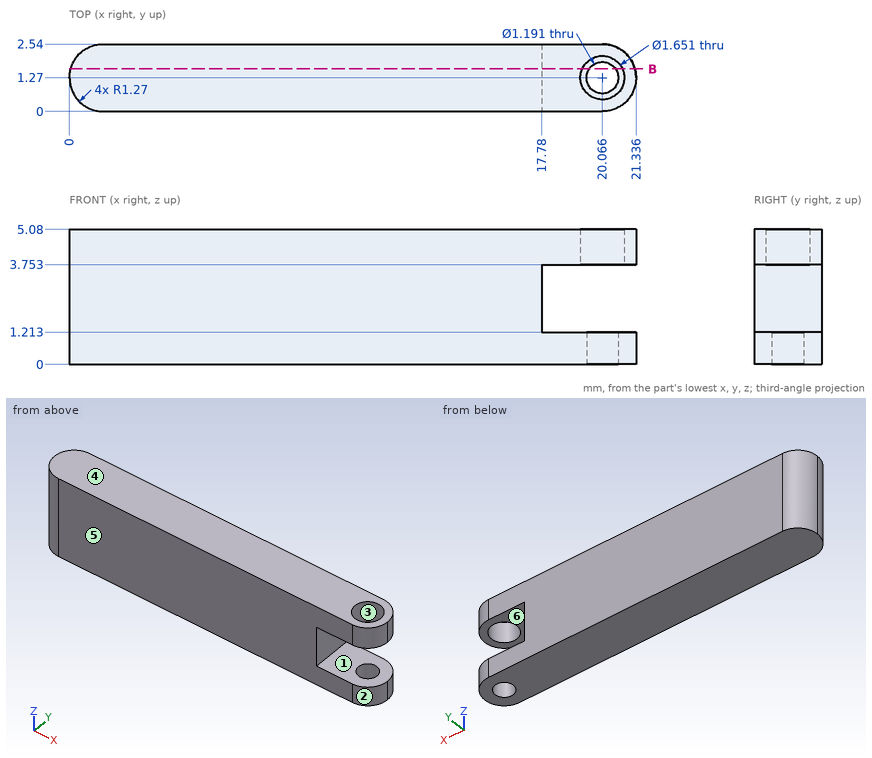
Geometry: see drawing. Coordinates: mm, zero at the bounding-box minimum. A direction names the side the tool comes from. Round coordinates to 2 decimals unless told otherwise and drop trailing zeros. Loops run counter-clockwise (first coordinate to the right, second up) from the corner with the lowest first, then second, coordinate; pieces in that order, holes last. Notation, with made-up numbers: (61, 72.5) -> (92, 72.5) arc R25 cw to (92, 86.5) -> close; hole circle Ø11 at (15, -24). An arc over 180 degrees is marked (long way). Use one line per item in the form item = value. Start each with the question number.
Item 1: Contact query for a flat-ended pin moving along its axis: pin 1 Ø0.8 at (y, z) = (2, 2.5) entering from +X. Output: stop coordinate, or through.
Item 2: Material intervals for L1, parallel to Z at x = 19, y = 0.75; L2, parallel to X at y = 1.35, z = 4.3 (1 decimal); L3, parallel to X at y = 1.7, z = 0.65 (1 decimal), sorted ascending. Write a range as from..to.
Item 3: Set-up query: the marked faces 1, 2 and 3. Return all of +Z, -Z, +X, -X, +Y, -Y with unobstructed straight access to the full face (end or side cutting, diameter ignored); none if empty.
Item 4: Section query B-B on y = 1.6. Return the cut outline in (x, z), then the cut area to 3 significant figures.
Item 5: Mould query, pull axis Z, two halves, no side actions, for the marked faces 4, 5 and 6. Classes: pulls with the +Z half, pulls with the -Z half, needs draft (parallel to the pull), parting line crosses it, or undercut.
Ans:
q1.pin_1 = 17.78
q2.L1 = 0..1.21, 3.75..5.08
q2.L2 = 0..19.2, 20.9..21.3
q2.L3 = 0.1..19.7, 20.5..21.3
q3.face_1 = +X, +Y, -Y
q3.face_2 = +Z, -Z, +X, -Y
q3.face_3 = +Z
q4.outline = (0.04, 0) -> (19.57, 0) -> (19.57, 1.21) -> (17.78, 1.21) -> (17.78, 3.75) -> (19.31, 3.75) -> (19.31, 5.08) -> (0.04, 5.08) -> close; (20.56, 0) -> (21.29, 0) -> (21.29, 1.21) -> (20.56, 1.21) -> close; (20.82, 3.75) -> (21.29, 3.75) -> (21.29, 5.08) -> (20.82, 5.08) -> close
q4.area = 95.8 mm^2
q5.face_4 = pulls with the +Z half
q5.face_5 = needs draft
q5.face_6 = undercut
